Work out the finished part from the listing and answer in its coordinate system (mm). A direction names the side the tool comes from. Give positions to 0.01 mm unless a question says otherwise; leave off trailing zeros. Loops run counter-clockwise (first coordinate to the right, second up) from the corner with the lowest first, then second, coordinate; pieces in that order, holes last.
```python
from build123d import *
from build123d.topology import SkipClean

# Parameters (mm, degrees)
BOSS_EXTRUDE1_DEPTH = 25
CUT_EXTRUDE1_DEPTH  = 148.978005832
CUT_EXTRUDE9_DEPTH  = 3
CUT_EXTRUDE10_START = -25
CUT_EXTRUDE10_DEPTH = 173.978005832
SKETCH6_3_R         = 12.5
CUT_EXTRUDE11_DEPTH = 148.978005832
BOSS_EXTRUDE2_START = 4
SKETCH7_R           = 28
SKETCH7_R_2         = 16
BOSS_EXTRUDE2_DEPTH = 18
LPATTERN1_COUNT     = 2
LPATTERN1_PITCH     = 52
BOSS_EXTRUDE3_DEPTH = 36
SKETCH9_R           = 12.5
CUT_EXTRUDE12_DEPTH = 168.010449404
CUT_EXTRUDE13_DEPTH = 168.426073866
CUT_EXTRUDE14_DEPTH = 3
LPATTERN2_COUNT     = 2
LPATTERN2_PITCH     = 45
SKETCH12_R          = 7.5
CUT_EXTRUDE15_DEPTH = 168.426073866


with BuildPart() as part:
    # Sketch2 → Boss-Extrude1 (new, symmetric)
    with BuildSketch(Plane.XY):
        Polygon((-1, -32.433962264), (31, -32.433962264), (31, 35.566037736), (9, 35.566037736), (9, 80.566037736), (12, 80.566037736), (12, 130.566037736), (0, 130.566037736), (-34, 130.566037736), (-34, 80.566037736), (-9, 80.566037736), (-9, 35.566037736), (-31, 35.566037736), (-31, -32.433962264), align=None)
    extrude(amount=BOSS_EXTRUDE1_DEPTH, both=True)

    # Sketch3 → Cut-Extrude1 (cut, through all)
    with BuildSketch(Plane(origin=(31, 0, 0), x_dir=(0, 0, -1), z_dir=(1, 0, 0))):
        with BuildLine():
            Line((-28, -4.433962264), (-30.641953589, -47.1115747))
            Line((-30.641953589, -47.1115747), (44.761332348, -47.1115747))
            Line((44.761332348, -47.1115747), (28, -4.433962264))
            ThreePointArc((28, -4.433962264), (0, 23.566037736), (-28, -4.433962264))
        make_face()
        with BuildLine():
            Line((-25, 105.566037736), (-43.623428006, 147.748377779))
            Line((-43.623428006, 147.748377779), (44.761332348, 142.473077281))
            Line((44.761332348, 142.473077281), (25, 105.566037736))
            ThreePointArc((25, 105.566037736), (0, 130.566037736), (-25, 105.566037736))
        make_face()
    extrude(amount=-CUT_EXTRUDE1_DEPTH, mode=Mode.SUBTRACT)

    # Sketch5 → Cut-Extrude9 (cut)
    with SkipClean():  # the faces are left unmerged after this step: merging them gives an invalid solid
        with BuildSketch(Plane(origin=(12, 0, 0), x_dir=(0, 0, -1), z_dir=(1, 0, 0))):
            with BuildLine():
                ThreePointArc((25, 105.566037736), (17.677669479, 87.888368155), (-1.45e-07, 80.566037736))
                Line((-1.45e-07, 80.566037736), (25, 80.566037736))
                Line((25, 80.566037736), (25, 105.566037736))
            make_face()
            with BuildLine():
                ThreePointArc((-1.45e-07, 80.566037736), (-17.677669581, 87.888368257), (-25, 105.566037736))
                Line((-25, 105.566037736), (-25, 80.566037736))
                Line((-25, 80.566037736), (-1.45e-07, 80.566037736))
            make_face()
        extrude(amount=-CUT_EXTRUDE9_DEPTH, mode=Mode.SUBTRACT)

    # Sketch6 → Cut-Extrude10 (cut, through all)
    with SkipClean():  # the faces are left unmerged after this step: merging them gives an invalid solid
        with BuildSketch(Plane.ZY.offset(34).offset(CUT_EXTRUDE10_START)):
            with BuildLine():
                Line((25, 80.566037736), (25, 105.566037736))
                ThreePointArc((25, 105.566037736), (17.6776695, 87.888368176), (-8.4e-08, 80.566037736))
                Line((-8.4e-08, 80.566037736), (25, 80.566037736))
            make_face()
            with BuildLine():
                ThreePointArc((-8.4e-08, 80.566037736), (-17.677669559, 87.888368236), (-25, 105.566037736))
                Line((-25, 105.566037736), (-25, 80.566037736))
                Line((-25, 80.566037736), (-8.4e-08, 80.566037736))
            make_face()
        extrude(amount=CUT_EXTRUDE10_DEPTH, mode=Mode.SUBTRACT)

    # Sketch6<3> → Cut-Extrude11 (cut, through all)
    with SkipClean():  # the faces are left unmerged after this step: merging them gives an invalid solid
        with BuildSketch(Plane.ZY.offset(34)):
            with Locations(Location((0, 105.566037736, 0), (0, 0, 270))):
                Circle(SKETCH6_3_R)
        extrude(amount=-CUT_EXTRUDE11_DEPTH, mode=Mode.SUBTRACT)

    # Sketch7 → Boss-Extrude2 (add)
    with SkipClean():  # the faces are left unmerged after this step: merging them gives an invalid solid
        with BuildSketch(Plane(origin=(31, 0, 0), x_dir=(0, 0, -1), z_dir=(1, 0, 0)).offset(BOSS_EXTRUDE2_START)):
            with Locations((0, -4.433962264)):
                Circle(SKETCH7_R)
            with Locations((0, -4.433962264)):
                Circle(SKETCH7_R_2, mode=Mode.SUBTRACT)
        boss_extrude2 = extrude(amount=-BOSS_EXTRUDE2_DEPTH)

    # LPattern1: Boss-Extrude2 ×2
    with SkipClean():  # the faces are left unmerged after this step: merging them gives an invalid solid
        with Locations(*[(-i * LPATTERN1_PITCH, 0, 0) for i in range(1, LPATTERN1_COUNT)]):
            add(boss_extrude2)

    # Sketch8 → Boss-Extrude3 (add)
    with SkipClean():  # the faces are left unmerged after this step: merging them gives an invalid solid
        with BuildSketch(Plane(origin=(0, 130.566037736, 0), x_dir=(1, 0, 0), z_dir=(0, 1, 0))):
            Polygon((-20, 0), (-2, 0), (-2, -30), (10, -30), (10, -42), (13, -42), (13, -78), (-2, -78), (-2, -42), (-20, -42), (-20, -78), (-35, -78), (-35, -42), (-32, -42), (-32, -30), (-20, -30), align=None)
        extrude(amount=-BOSS_EXTRUDE3_DEPTH)

    # Sketch9 → Cut-Extrude12 (cut, through all)
    with SkipClean():  # the faces are left unmerged after this step: merging them gives an invalid solid
        with BuildSketch(Plane.ZY.offset(34)):
            with Locations(Location((0, 105.566037736, 0), (0, 0, 270))):
                Circle(SKETCH9_R)
        extrude(amount=-CUT_EXTRUDE12_DEPTH, mode=Mode.SUBTRACT)

    # Sketch10 → Cut-Extrude13 (cut, through all)
    with SkipClean():  # the faces are left unmerged after this step: merging them gives an invalid solid
        with BuildSketch(Plane.ZY.offset(35)):
            with BuildLine():
                Line((60, 94.566037736), (99.579352657, 93.222301479))
                Line((99.579352657, 93.222301479), (99.579352657, 133.580048743))
                Line((99.579352657, 133.580048743), (60, 130.566037736))
                ThreePointArc((60, 130.566037736), (78, 112.566037736), (60, 94.566037736))
            make_face()
        extrude(amount=-CUT_EXTRUDE13_DEPTH, mode=Mode.SUBTRACT)

    # Sketch11 → Cut-Extrude14 (cut)
    with SkipClean():  # the faces are left unmerged after this step: merging them gives an invalid solid
        with BuildSketch(Plane.ZY.offset(35)):
            with BuildLine():
                Line((60, 130.566037736), (34.988350442, 136.05842118))
                Line((34.988350442, 136.05842118), (42, 90.490327212))
                Line((42, 90.490327212), (60, 94.566037736))
                ThreePointArc((60, 94.566037736), (42, 112.566037736), (60, 130.566037736))
            make_face()
        cut_extrude14 = extrude(amount=-CUT_EXTRUDE14_DEPTH, mode=Mode.SUBTRACT)

    # LPattern2: Cut-Extrude14 ×2
    with SkipClean():  # the faces are left unmerged after this step: merging them gives an invalid solid
        with Locations(*[(i * LPATTERN2_PITCH, 0, 0) for i in range(1, LPATTERN2_COUNT)]):
            add(cut_extrude14, mode=Mode.SUBTRACT)

    # Sketch12 → Cut-Extrude15 (cut, through all)
    with SkipClean():  # the faces are left unmerged after this step: merging them gives an invalid solid
        with BuildSketch(Plane.ZY.offset(35)):
            with Locations((60, 112.566037736)):
                Circle(SKETCH12_R)
        extrude(amount=-CUT_EXTRUDE15_DEPTH, mode=Mode.SUBTRACT)


solid = part.part
```
Q1. Section C-C on y = 19 is taken. Give the vertices of the cut face in (x, z), plus the area to 3 significant figures.
Q2. Section A-A on y = 1 is taken. Give the vertices of the cut face in (x, z), plus the area to 3 significant figures.
Q3. Consider line 1 along Y through (x, z) = (2, 60); line 2 along X through (y, z) = (95.5, 53); line 3 along Y through (x, z) = (23, 0). Determine where each line is inside the solid, lowest interval first.
Q4. Section B-B on x = 6 is taken. Give the vertices of the cut face in (y, z), plus the area to 3 significant figures.
Q5. Which of the six approach directions +Z, -Z, +X, -X, +Y, -Y give full straight-line access (tool end or side, diameter ignored) to faces 1 (the face through (4, 113, 30)), 2 (the face through (-29.272, 110.223, 77.847)), 3 (the face through (-20, 113, 52))?
Q6. Determine the mould class of faces 4 (the face through (0.238, 23.563, -0.433)), 5 (the face through (-11, 94.566, 41)), 6 (the face through (0, 47, -25)) for opening direction Z: +Z half, -Z half, draft (parallel to the pull), parting line (faces both ways), or undercut.
Q7. Given pin 1 (1 mm diameter, centred on x = -7.5, y = 48, fed in from +Z); pin 2 (9 mm diameter, centred on y = 117, z = 40, fed in from -X); pin 3 (9.5 mm diameter, centred on x = 1.5, y = 106.5, fed in from -Z); pin 4 (10 mm diameter, centred on x = -9, z = -8, fed in from +Y), each flat-ended and moving along its own axis, determine where each tip first touches the part or whether it passes through.
Q8. Section D-D on y = 89 is taken. Give the vertices of the cut face in (x, z), plus the area to 3 significant figures.
Check result:
1. outline: (-35, -15.32) - (-31, -15.32) - (-31, -25) - (31, -25) - (31, -15.32) - (35, -15.32) - (35, 15.32) - (31, 15.32) - (31, 25) - (-31, 25) - (-31, 15.32) - (-35, 15.32) - close; hole (-17, -15.32) - (17, -15.32) - (17, 15.32) - (-17, 15.32) - close
1. area: 2,300 mm2
2. outline: (-35, -27.47) - (-17, -27.47) - (-17, -15.05) - (-35, -15.05) - close; (-35, 15.05) - (-17, 15.05) - (-17, 27.47) - (-35, 27.47) - close; (17, -27.47) - (35, -27.47) - (35, -15.05) - (17, -15.05) - close; (17, 15.05) - (35, 15.05) - (35, 27.47) - (17, 27.47) - close
2. area: 894 mm2
3. line 1: y = 94.57 to 105.07, 120.07 to 130.57
3. line 2: x = -32 to -20, -2 to 10
3. line 3: y = -32.43 to -20.43, 11.57 to 35.57
4. outline: (8.18, -25) - (105.57, -25) arc R25 ccw to (105.57, 25) - (8.18, 25) arc R28 cw to start; (94.57, 30) - (130.57, 30) - (130.57, 60) arc R18 ccw to (94.57, 60) - close; hole circle Ø25 at (105.57, 0); hole circle Ø15 at (112.57, 60)
4. area: 6,220 mm2
5. face 1: +X, +Y, -Y
5. face 2: -X
5. face 3: +Z, +Y, -Y
6. face 4: undercut
6. face 5: draft
6. face 6: -Z half
7. pin 1: stops at z = 25
7. pin 2: stops at x = -35
7. pin 3: stops at z = -25
7. pin 4: stops at y = 130.39
8. outline: (-34, -18.72) - (-9, -18.72) - (-9, -25) - (9, -25) - (9, -18.72) - (12, -18.72) - (12, 18.72) - (9, 18.72) - (9, 25) - (-9, 25) - (-9, 18.72) - (-34, 18.72) - close
8. area: 1,950 mm2
